Read the model definition and answer for the solid it produces. Units are mm, in the model's axes. Face numbers are marked on the shaded views. A direction names the side the tool comes from. Coordinates: 2 decimals unless noted, no trailing zeros. Loops run counter-clockwise (first coordinate to the right, second up) from the corner with the lowest first, then second, coordinate; pieces in that order, holes last.
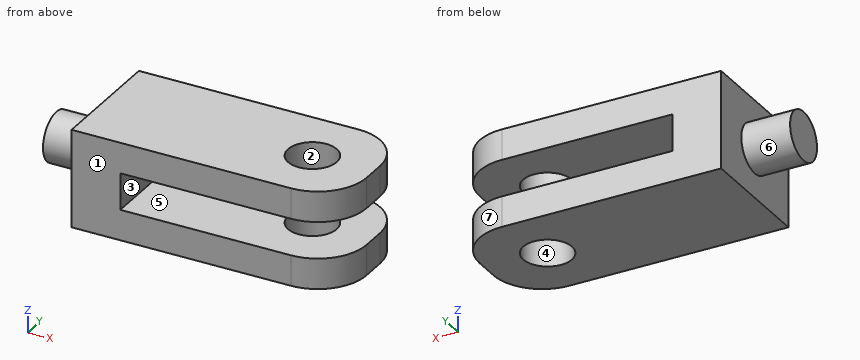
from build123d import *

# Parameters (mm, degrees)
SKETCH1_W           = 165
SKETCH1_H           = 75
BOSS_EXTRUDE1_DEPTH = 60
SKETCH2_W           = 22.5
SKETCH2_H           = 75
CUT_EXTRUDE1_DEPTH  = 135
FILLET1_R           = 30
SKETCH3_R           = 15
CUT_EXTRUDE2_DEPTH  = 109.685325596
SKETCH4_R           = 15
BOSS_EXTRUDE2_DEPTH = 30


with BuildPart() as part:
    # Sketch1 → Boss-Extrude1 (new body)
    with BuildSketch(Plane.XY):
        Rectangle(SKETCH1_W, SKETCH1_H)
    extrude(amount=BOSS_EXTRUDE1_DEPTH)

    # Sketch2 → Cut-Extrude1 (cut)
    with BuildSketch(Plane(origin=(82.5, 0, 0), x_dir=(0, 0, -1), z_dir=(1, 0, 0))):
        with Locations((-30, 0)):
            Rectangle(SKETCH2_W, SKETCH2_H)
    extrude(amount=-CUT_EXTRUDE1_DEPTH, mode=Mode.SUBTRACT)

    # Fillet1
    fillet1_edges = [part.edges().sort_by_distance(p)[0] for p in [
        (82.5, -37.5, 9.375),
        (82.5, 37.5, 9.375),
        (82.5, 37.5, 50.625),
        (82.5, -37.5, 50.625),
    ]]
    fillet(fillet1_edges, radius=FILLET1_R)

    # Sketch3 → Cut-Extrude2 (cut, through all)
    with BuildSketch(Plane.XY.offset(60)):
        with Locations((45, 0)):
            Circle(SKETCH3_R)
    extrude(amount=-CUT_EXTRUDE2_DEPTH, mode=Mode.SUBTRACT)

    # Sketch4 → Boss-Extrude2 (add)
    with BuildSketch(Plane.ZY.offset(82.5)):
        with Locations(Location((30, 0, 0), (0, 0, 180))):
            Circle(SKETCH4_R)
    extrude(amount=BOSS_EXTRUDE2_DEPTH)


solid = part.part
Q1. A cutting plane is placed at D-D (z = 54). Give the vertices of the cut face in (x, y), then the cut area to 3 significant figures.
Findings below:
outline: (-82.5, -37.5) - (52.5, -37.5) arc R30 ccw to (82.5, -7.5) - (82.5, 7.5) arc R30 ccw to (52.5, 37.5) - (-82.5, 37.5) - close; hole circle Ø30 at (45, 0)
area: 11,300 mm2
Q2. A cutting plane is placed at B-B (y = 0). Give the vertices of the cut face in (x, z).
Findings below:
outline: (-112.5, 15) - (-82.5, 15) - (-82.5, 0) - (30, 0) - (30, 18.75) - (-52.5, 18.75) - (-52.5, 41.25) - (30, 41.25) - (30, 60) - (-82.5, 60) - (-82.5, 45) - (-112.5, 45) - close; (60, 0) - (82.5, 0) - (82.5, 18.75) - (60, 18.75) - close; (60, 41.25) - (82.5, 41.25) - (82.5, 60) - (60, 60) - close
Q3. A cutting plane is placed at A-A (x = 19). Give the vertices of the cut face in (y, z), then the cut area to 3 significant figures.
Findings below:
outline: (-37.5, 0) - (37.5, 0) - (37.5, 18.75) - (-37.5, 18.75) - close; (-37.5, 41.25) - (37.5, 41.25) - (37.5, 60) - (-37.5, 60) - close
area: 2,810 mm2
Q4. Straight lines are drawn through the part: probe 1 along Z at (x, y) = (-48.5, -1.5); probe 2 along Y at (x, z) = (45, 12); probe 3 along Z at (x, y) = (-100, 0.5). For each, find the intervals that lie inside material, in ascending order.
Findings below:
probe 1: z = 0 to 18.75, 41.25 to 60
probe 2: y = -37.5 to -15, 15 to 37.5
probe 3: z = 15.01 to 44.99
Q5. A cutting plane is placed at C-C (x = 45). Give the vertices of the cut face in (y, z), then the cut area to 3 significant figures.
Findings below:
outline: (-37.5, 0) - (-15, 0) - (-15, 18.75) - (-37.5, 18.75) - close; (-37.5, 41.25) - (-15, 41.25) - (-15, 60) - (-37.5, 60) - close; (15, 0) - (37.5, 0) - (37.5, 18.75) - (15, 18.75) - close; (15, 41.25) - (37.5, 41.25) - (37.5, 60) - (15, 60) - close
area: 1,690 mm2
Q6. Which of the six approach directions +Z, -Z, +X, -X, +Y, -Y give full straight-line access (tool end or side, diameter ignored) to the marked faces 5, 6 and 7?
Findings below:
face 5: +X, +Y, -Y
face 6: -X
face 7: +Z, -Z, +X, +Y
Q7. Determine the mould class of the marked faces 1, 2, 3 and 4 for opening direction X: +X half, -X half, draft (parallel to the pull), parting line (faces both ways), or undercut.
Findings below:
face 1: draft
face 2: undercut
face 3: +X half
face 4: undercut
Q8. Flat-ended cylindrical pins translate along their axes: pin 1 Ø1.5 at (y, z) = (-17.5, 45.5) entering from -X; pin 2 Ø25 at (y, z) = (-9.5, 31.5) entering from +X. Find the tip coordinate at first contact, or state that the pin passes through.
Findings below:
pin 1: stops at x = -82.5
pin 2: stops at x = 82.5
